Model file for the job. Use its own axes, mm. A direction names the side the tool comes from. Coordinates: 2 decimals unless noted, no trailing zeros. Order: outer loops, then holes, each group sorted by start corner. A loop starts at its lowest first (then second) coordinate and runs counter-clockwise, first axis right, second up. Notation, with made-up numbers: (85.25, 13) -> (101.25, 13) arc R25 ccw to (101.25, 52) -> close; hole circle Ø10 at (88.5, 52.5). An arc over 180 degrees is marked (long way). Use CSV: the item, a comma, the result in double quotes. Start each with the question number.
(1) Cut at A-A on x = -21. Write the cut outline in (y, z), plus the area to 3 significant figures.
(2) Probe L1, parallel to X at y = -1.3, z = -2.5; L2, parallel to Z at x = -23, y = -1.05; L3, parallel to Z at x = 17.5, y = -1.2. List the from-to ranges inside material, lowest first.
(3) Cut at C-C on z = 16. Write the cut outline in (x, y), plus the area to 3 significant figures.
(4) Cut at B-B on x = 17.5. Write the cut outline in (y, z).
(5) Tool access for faces 1 (the flat face through (-14, 0, -1.65)), 2 (the flat face through (16.3, 0, 2)), 3 (the flat face through (14, 0, 1.65)), 4 (the flat face through (-22.5, 0, 16)), 5 (the flat face through (0, 1.5, 0)): list every direction of +Z, -Z, +X, -X, +Y, -Y with a clear straight run to the whole face (end or side of a thin tool).
(6) Pin check, flat tips, straight feed: pin 1 Ø1 at (y, z) = (1, 16.5) entering from -X; pin 2 Ø1.5 at (x, y) = (-24, 0.5) entering from +Z; pin 3 Ø1.5 at (x, y) = (-24.5, 0.5) entering from -Z. Stop position of each tip, or through.
(7) Cut at D-D on z = -1. Write the cut outline in (x, y).
(8) Pull direction X, two halves, no side cores. Call faces 6 (the flat face through (-12.5, 0, 0)), 7 (the flat face through (-14, 0, 1.65)), 8 (the flat face through (-19.5, 0, 2)): pulls with the +X half, pulls with the -X half, needs draft (parallel to the pull), parting line crosses it, or undercut.
```python
from build123d import *

# Parameters (mm, degrees)
SKETCH_1_W          = 45
SKETCH_1_H          = 50
SKETCH_1_W_2        = 3
SKETCH_1_H_2        = 15
EXTRUDE_1_DEPTH     = 1.5
SKETCH_2_W          = 3.8
SKETCH_2_H          = 3.3
SKETCH_2_W_2        = 3.2
SKETCH_2_H_2        = 1.45
SKETCH_2_W_3        = 6
CUT_EXTRUDE_1_DEPTH = 36.836433974


with BuildPart() as part:
    # 草图1 → 凸台-拉伸1 (new, symmetric)
    with BuildSketch(Plane(origin=(0, 0, 0), x_dir=(1, 0, 0), z_dir=(0, 1, 0))):
        Rectangle(SKETCH_1_W, SKETCH_1_H)
        with Locations((-24, 0)):
            Rectangle(SKETCH_1_W_2, SKETCH_1_H_2)
        with Locations((24, 0)):
            Rectangle(SKETCH_1_W_2, SKETCH_1_H_2)
    extrude(amount=EXTRUDE_1_DEPTH, both=True)

    # 草图2 → 切除-拉伸1 (cut, symmetric)
    with BuildSketch(Plane(origin=(0, 1.5, 0), x_dir=(1, 0, 0), z_dir=(0, 1, 0))):
        with Locations((14.4, 0)):
            Rectangle(SKETCH_2_W, SKETCH_2_H)
        with Locations((17.9, 2.375)):
            Rectangle(SKETCH_2_W_2, SKETCH_2_H_2)
        with Locations((17.9, 0)):
            Rectangle(SKETCH_2_W_2, SKETCH_2_H)
        with Locations((17.9, -2.375)):
            Rectangle(SKETCH_2_W_2, SKETCH_2_H_2)
        with Locations((22.5, 0)):
            Rectangle(SKETCH_2_W_3, SKETCH_2_H)
    cut_extrude_1 = extrude(amount=CUT_EXTRUDE_1_DEPTH, both=True, mode=Mode.SUBTRACT)

    # 镜向1: 切除-拉伸1 across plane
    add(cut_extrude_1.mirror(Plane(origin=(0, 0, 0), x_dir=(0, 0, 1), z_dir=(1, 0, 0))), mode=Mode.SUBTRACT)


solid = part.part
```
Outcome:
1,outline,"(-1.5, -25) -> (1.5, -25) -> (1.5, -1.65) -> (-1.5, -1.65) -> close; (-1.5, 1.65) -> (1.5, 1.65) -> (1.5, 25) -> (-1.5, 25) -> close"
1,area,"140 mm2"
2,L1,"-25.5 to -19.5, -16.3 to 16.3, 19.5 to 25.5"
2,L2,"-7.5 to -1.65, 1.65 to 7.5"
2,L3,"-25 to -3.1, 3.1 to 25"
3,outline,"(-22.5, -1.5) -> (22.5, -1.5) -> (22.5, 1.5) -> (-22.5, 1.5) -> close"
3,area,"135 mm2"
4,outline,"(-1.5, -25) -> (1.5, -25) -> (1.5, -3.1) -> (-1.5, -3.1) -> close; (-1.5, 3.1) -> (1.5, 3.1) -> (1.5, 25) -> (-1.5, 25) -> close"
5,face 1,"-X, +Y, -Y"
5,face 2,"+Y, -Y"
5,face 3,"+X, +Y, -Y"
5,face 4,"+Z, -X, +Y, -Y"
5,face 5,"+Z, -Z, +X, -X, +Y"
6,pin 1,"x = -22.5"
6,pin 2,"z = 7.5"
6,pin 3,"z = -7.5"
7,outline,"(-12.5, -1.5) -> (12.5, -1.5) -> (12.5, 1.5) -> (-12.5, 1.5) -> close"
8,face 6,"pulls with the -X half"
8,face 7,"needs draft"
8,face 8,"undercut"
